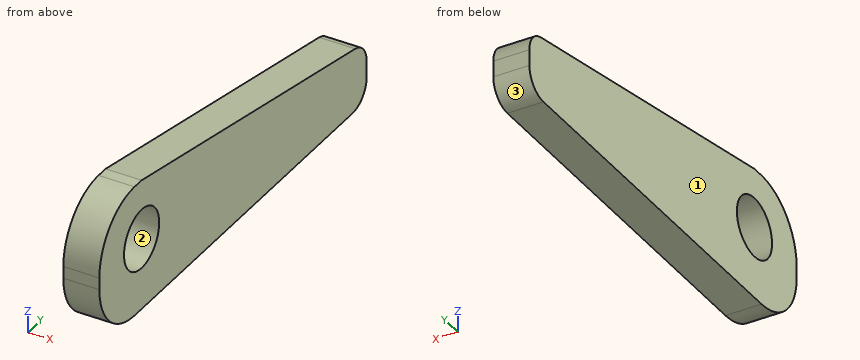
```python
from build123d import *

# Parameters (mm, degrees)
F0_R     = 2.5
F1_DEPTH = 3
F2_R     = 2
F3_R     = 5
F4_R     = 2


with BuildPart() as f1:
    # F0 (on Right) → F1 (new body)
    with BuildSketch(Plane.YZ):
        Polygon((-19, 11), (-19, 0), (19, 0), (19, 5), (-13, 11), align=None)
        with Locations((-13, 6)):
            Circle(F0_R, mode=Mode.SUBTRACT)
    extrude(amount=F1_DEPTH)

    # F2
    f2_edges = [f1.edges().sort_by_distance(p)[0] for p in [
        (1.5, 19, 0),
    ]]
    fillet(f2_edges, radius=F2_R)

    # F3
    f3_edges = [f1.edges().sort_by_distance(p)[0] for p in [
        (1.5, -19, 11),
        (1.5, -19, 0),
    ]]
    fillet(f3_edges, radius=F3_R)

    # F4
    f4_edges = [f1.edges().sort_by_distance(p)[0] for p in [
        (1.5, 19, 5),
    ]]
    fillet(f4_edges, radius=F4_R)


solid = f1.part
```
Design review of the part built by this model. Coordinates are the model's own, in mm. Face numbers are marked on the shaded views. Give positions to 0.01 mm unless a question says otherwise; leave off trailing zeros. Order: outer loops, then holes, each group sorted by start corner. A loop starts at its lowest first (then second) coordinate and runs counter-clockwise, first axis right, second up. Notation, with made-up numbers: M 84.25,1 L 121.25,1 A16 cw 121.25,5 Z; hole C -25.75,-12 d1. An arc over 180 degrees is marked long. One line per question, with ' | ' between items. Start each with the question number.
Q1. For L1, parallel to Z at x = 1.15, y = -13; L2, parallel to Y at x = 1.3, z = 4.75; L3, parallel to Z at x = 0.55, y = -2, list the stretches that pass through material, from the lowest coordinate up. Write a range as [from, to].
Q2. We need section A-A (x = 1.15). Write out the cut boundary in (y, z), plus the area to 3 significant figures.
Q3. We need section D-D (y = 1.5). Write out the cut boundary in (x, z).
Q4. We need section C-C (z = 4.25). Write out the cut boundary in (x, y), plus the area to 3 significant figures.
Q5. We need section B-B (z = 6.5). Write out the cut boundary in (x, y), plus the area to 3 significant figures.
Q6. The part is to be moulded in two halves that separate along Z. For the marked faces 1, 2 and 3, say which applies: +Z half, -Z half, draft (parallel to the pull), parting line (faces both ways), or undercut.
Q7. For pin 1 Ø4 at (y, z) = (-13, 6) entering from +X; pin 2 Ø1.5 at (x, z) = (1, 9) entering from -Y; pin 3 Ø4 at (y, z) = (2, 7) entering from -X, all flat-tipped, find the tip position at first contact; note any pin that passes through.
Returned:
1) L1: [0, 3.5], [8.5, 11] | L2: [-18.99, -15.17], [-10.83, 18.42] | L3: [0, 8.94]
2) outline: M -19,5 A5 ccw -14,0 L 17,0 A2 ccw 19,2 L 19,3.34 A2 ccw 17.37,5.31 L -13,11 L -14,11 A5 ccw -19,6 Z; hole C -13,6 d5 | area: 290 mm2
3) outline: M 0,0 L 3,0 L 3,8.28 L 0,8.28 Z
4) outline: M 0,-18.94 L 3,-18.94 L 3,-14.79 L 0,-14.79 Z; M 0,-11.21 L 3,-11.21 L 3,18.78 L 0,18.78 Z | area: 102 mm2
5) outline: M 0,-18.97 L 3,-18.97 L 3,-15.45 L 0,-15.45 Z; M 0,-10.55 L 3,-10.55 L 3,11 L 0,11 Z | area: 75.2 mm2
6) face 1: draft | face 2: undercut | face 3: -Z half
7) pin 1: through | pin 2: y = -18.47 | pin 3: x = 0
